Part print with two shaded views. Sizes in mm from the minimum x, y, z corner. A direction names the side the tool comes from. Give positions to 0.01 mm unless a question says otherwise; leave off trailing zeros. Order: outer loops, then holes, each group sorted by start corner. A loop starts at its lowest first (then second) coordinate and runs counter-clockwise, first axis right, second up. Notation, with made-up numbers: M 24.25,57 L 68.25,57 A23 cw 68.25,74 Z; hole C 77,46.25 d10. An arc over 180 degrees is marked long. Return JSON: item names as keys, results as strings. Group by question number.
1. Pin check, flat tips, straight feed: pin 1 (4 mm diameter, centred on x = 18.5, z = 4.5, fed in from +Y); pin 2 (3 mm diameter, centred on x = 7.5, z = 17, fed in from +Y); pin 3 (4 mm diameter, centred on x = 6, z = 4.5, fed in from +Y). Stop position of each tip, or through.
2. Two-plate mould, pull along Z, no slides. Class the marked faces 4, 5 and 6: released by +Z, released by -Z, zero draft, split by the parting line, or undercut.
3. Slice it at D-D on x = 15.5. List the corners of the cut face in (y, z) (3 decimals).
4. Wall check: probe 1 along Y at (x, z) = (9.75, 12.7) (3 decimals); probe 2 along Z at (x, y) = (11.5, 12.5); probe 3 along Y at (x, z) = (17, 12.7). Give the ranges that are in metal, low to high. Write a range as [from, to].
5. Slice it at C-C on x = 7.25. List the corners of the cut face in (y, z).
6. 3-axis set-ups, long thin cutter, end or side, ignore diameter. For the marked faces 1, 2 and 3: which of +Z, -Z, +X, -X, +Y, -Y reach the whole face in a straight line?
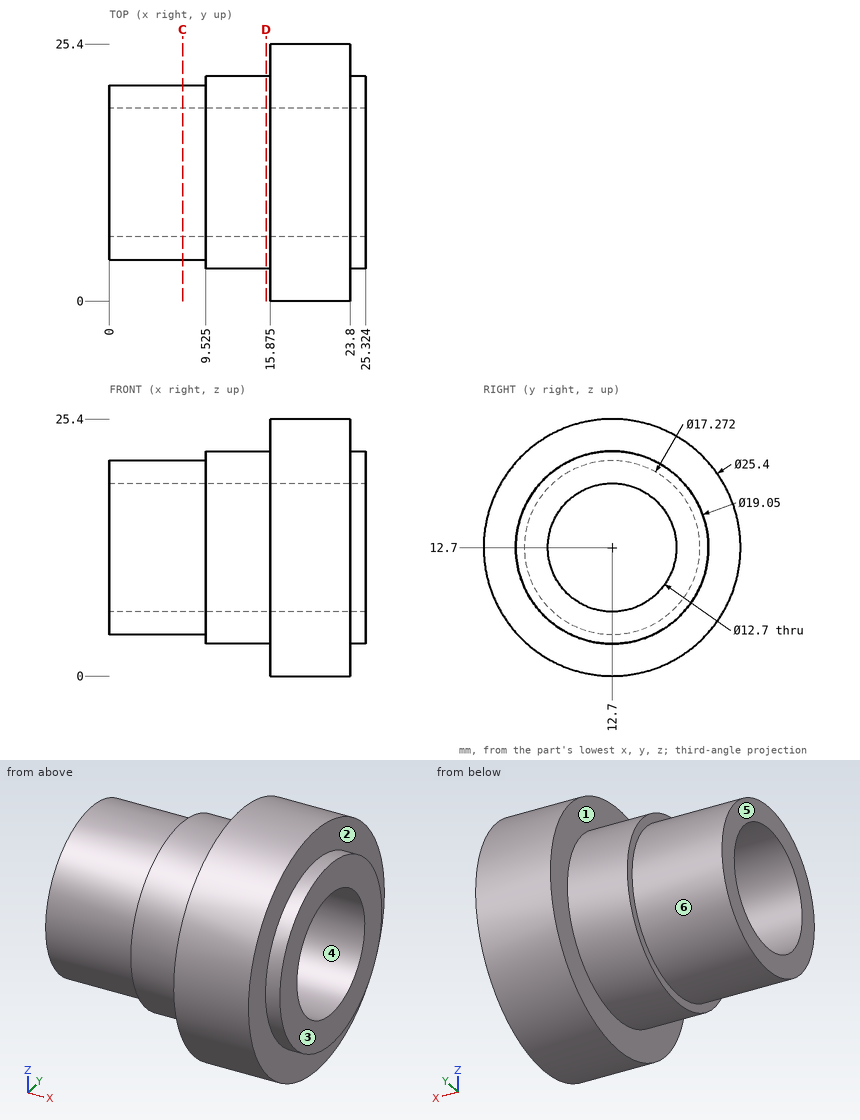
Result:
{
 "1": {"pin 1": "stops at y = 23.78", "pin 2": "stops at y = 20.87", "pin 3": "stops at y = 18.71"},
 "2": {"face 4": "undercut", "face 5": "zero draft", "face 6": "split by the parting line"},
 "3": {"outline": "C 12.7,12.7 d19.05; hole C 12.7,12.7 d12.7"},
 "4": {"probe 1": "y = [3.175, 6.35], [19.05, 22.225]", "probe 2": "z = [3.18, 6.35], [19.05, 22.22]", "probe 3": "y = [0, 6.35], [19.05, 25.4]"},
 "5": {"outline": "C 12.7,12.7 d17.27; hole C 12.7,12.7 d12.7"},
 "6": {"face 1": "-X", "face 2": "+X", "face 3": "+Z, -Z, +X, +Y, -Y"}
}
